Autodesk Inventor part; units mm, degrees
ref_plane "YZ Plane" through (0, 0, 0) normal (1, 0, 0) x (0, 1, 0)
ref_plane "XZ Plane" through (0, 0, 0) normal (0, 1, 0) x (-1, 0, 0)
ref_plane "XY Plane" through (0, 0, 0) normal (0, 0, 1) x (1, 0, 0)
sketch "Sketch1" plane through (0, 0, 0) normal (0, 0, 1) x (1, 0, 0)
  line L0 (122, -13.5) -> (-122, -13.5)
  line L1 (-122, -13.5) -> (-122, 13.5)
  line L2 (-122, 13.5) -> (122, 13.5)
  line L3 (122, 13.5) -> (122, -13.5)
  line L4 (122, -13.5) -> (-122, 13.5) construction
  line L5 (-122, -13.5) -> (122, 13.5) construction
  line L6 (0, 0) -> (-31, 0) construction
  circle A0 centre (-93, 0) radius 1.4
  circle A1 centre (-62, 0) radius 1.4
  circle A2 centre (-31, 0) radius 1.4
  circle A3 centre (0, 0) radius 1.4
  circle A4 centre (31, 0) radius 1.4
  circle A5 centre (62, 0) radius 1.4
  circle A6 centre (93, 0) radius 1.4
  dimension "d0" = 27
  dimension "d1" = 244
  dimension "d2" = 2.8
  dimension "d5" = 31
  dimension "d10" = 31
extrude "Extrusion1" add sketch "Sketch1" along normal blind 2 contours L0 L1 L2 L3 | A3
sketch "Sketch2" plane through (0, 0, 2) normal (0, 0, 1) x (1, 0, 0)
  line L0 (-5, 99.1699) -> (-5, 0)
  line L1 (-5, 0) -> (5, 0)
  line L2 (5, 0) -> (5, -99.1699)
  line L3 (232.2267, -99.1699) -> (-232.2267, -99.1699)
  line L4 (-232.2267, -99.1699) -> (-232.2267, 99.1699)
  line L5 (-232.2267, 99.1699) -> (232.2267, 99.1699)
  line L6 (232.2267, 99.1699) -> (232.2267, -99.1699)
  line L7 (232.2267, -99.1699) -> (-232.2267, 99.1699) construction
  line L8 (-232.2267, -99.1699) -> (232.2267, 99.1699) construction
  point P0 (0, 0)
  dimension "d13" = 10
extrude "Extrusion2" cut sketch "Sketch2" against normal through all contours L5 L6 L3 L2 L1 L0
properties part number "SensorLid"
Design review of the part built by this model. Coordinates are the model's own, in mm. A direction names the side the tool comes from. Coordinates: 2 decimals unless noted, no trailing zeros. Order: outer loops, then holes, each group sorted by start corner. A loop starts at its lowest first (then second) coordinate and runs counter-clockwise, first axis right, second up. Notation, with made-up numbers: (78, -26.5) -> (123, -26.5) arc R22 cw to (123, -7.5) -> close; hole circle Ø4 at (5.5, -13.75). An arc over 180 degrees is marked (long way). Use one line per item in the form item = value. Start each with the question number.
(1) Insertion check: pin 1 (0.6 mm diameter, centred on y = 6, z = 0.5, fed in from +X); pin 2 (1 mm diameter, centred on x = 0.5, z = 1, fed in from +Y). Each pin has a flat end and moves straight along its axis. Give the tip position at first contact, or say it passes through.
(2) For probe 1 along Y at (x, z) = (-93, 0.8); probe 2 along X at (y, z) = (4.25, 0.5); probe 3 along Y at (x, z) = (-62.5, 1.55), list the stretches that pass through material, from the lowest coordinate up.
(3) Add section C-C on y = 4.25. State the section outline as (x, z) points.
(4) For faces 1 (the cylindrical face through (-60.665, -0.421, 0.986)), 2 (the flat face through (-5, 7, 1)), list the 3-axis set-ups (+Z, -Z, +X, -X, +Y, -Y) from which the entire face can be reached by the end or side of a thin tool; tool diameter is ignored.
(5) Add section B-B on z = 1.1. State the section outline as (x, y) points, plus the area to 3 significant figures.
(6) The part is to be moulded in two halves that separate along X. For faces 3 (the cylindrical face through (-32.4, -0.06, 0.99)), 4 (the flat face through (-58, -13.5, 1)), 5 (the flat face through (-122, 0, 1)), say which applies: +X half, -X half, draft (parallel to the pull), parting line (faces both ways), or undercut.
(7) Add section A-A on x = -62. State the section outline as (y, z) points, plus the area to 3 significant figures.
Answer block:
q1.pin_1 = -5
q1.pin_2 = 0
q2.probe_1 = -13.5 to -1.4, 1.4 to 13.5
q2.probe_2 = -122 to -5
q2.probe_3 = -13.5 to -1.31, 1.31 to 13.5
q3.outline = (-122, 0) -> (-5, 0) -> (-5, 2) -> (-122, 2) -> close
q4.face_1 = +Z, -Z
q4.face_2 = +Z, -Z, +X, +Y
q5.outline = (-122, -13.5) -> (5, -13.5) -> (5, 0) -> (-5, 0) -> (-5, 13.5) -> (-122, 13.5) -> close; hole circle Ø2.8 at (-93, 0); hole circle Ø2.8 at (-62, 0); hole circle Ø2.8 at (-31, 0)
q5.area = 3,280 mm²
q6.face_3 = undercut
q6.face_4 = draft
q6.face_5 = -X half
q7.outline = (-13.5, 0) -> (-1.4, 0) -> (-1.4, 2) -> (-13.5, 2) -> close; (1.4, 0) -> (13.5, 0) -> (13.5, 2) -> (1.4, 2) -> close
q7.area = 48.4 mm²
